from build123d import *

# Parameters (mm, degrees)
SKETCH3_R                = 1.1811
BOSS_EXTRUDE1_DEPTH      = 0.7874
BOSS_EXTRUDE1_DEPTH_BACK = 0.7874
CUT_EXTRUDE1_DEPTH       = 1.7874


with BuildPart() as part:
    # Sketch3 → Boss-Extrude1 (new body, two sides)
    with BuildSketch(Plane.XY) as boss_extrude1_sk:
        with BuildLine():
            Line((-7.084786794, -26.251475436), (-5.5626, -20.611270532))
            Line((-5.5626, -20.611270532), (-9.244241607, -19.243466133))
            ThreePointArc((-9.244241607, -19.243466133), (-11.503586026, -21.079506525), (-14.357593282, -20.504768227))
            ThreePointArc((-14.357593282, -20.504768227), (0, 22.8727), (14.357593282, -20.504768227))
            ThreePointArc((14.357593282, -20.504768227), (11.503586026, -21.079506525), (9.244241607, -19.243466133))
            Line((9.244241607, -19.243466133), (5.5626, -20.611270532))
            Line((5.5626, -20.611270532), (7.084786794, -26.251475436))
            ThreePointArc((7.084786794, -26.251475436), (0, 27.1907), (-7.084786794, -26.251475436))
        make_face()
        with Locations((-7.986421892, -21.496599331)):
            Circle(SKETCH3_R, mode=Mode.SUBTRACT)
        with Locations((7.986421892, -21.496599331)):
            Circle(SKETCH3_R, mode=Mode.SUBTRACT)
    extrude(amount=BOSS_EXTRUDE1_DEPTH)
    extrude(boss_extrude1_sk.sketch, amount=-BOSS_EXTRUDE1_DEPTH_BACK)

    # Sketch4 → Cut-Extrude1 (cut, symmetric)
    with BuildSketch(Plane.XY):
        with BuildLine():
            Line((-7.395614895, -26.165608092), (-7.395614895, -33.561222987))
            Line((-7.395614895, -33.561222987), (0, -33.561222987))
            Line((0, -33.561222987), (0, -27.1907))
            Line((0, -27.1907), (0, -20.522811972))
            Line((0, -20.522811972), (-5.800698894, -20.522811972))
            ThreePointArc((-5.800698894, -20.522811972), (-6.322313955, -23.422176045), (-7.395614895, -26.165608092))
        make_face()
    cut_extrude1 = extrude(amount=CUT_EXTRUDE1_DEPTH, both=True, mode=Mode.SUBTRACT)

    # Mirror1: Cut-Extrude1 across plane
    add(cut_extrude1.mirror(Plane(origin=(0, 0, 0), x_dir=(0, 0, 1), z_dir=(1, 0, 0))), mode=Mode.SUBTRACT)


solid = part.part
Could you check a few things on this model? Use its own coordinates, in mm. A direction names the side the tool comes from. Give positions to 0.01 mm unless a question says otherwise; leave off trailing zeros. Order: outer loops, then holes, each group sorted by start corner. A loop starts at its lowest first (then second) coordinate and runs counter-clockwise, first axis right, second up. Notation, with made-up numbers: M 48,-36.5 L 59,-36.5 A30 cw 59,2.5 Z; hole C -2,72.25 d8. An arc over 180 degrees is marked long. One line per question, with ' | ' between items.
1. I want a section at C-C (z = -0.45). List the corners of the cut face in (x, y) for me.
Results:
outline: M -14.36,-20.5 A24.06 cw long 14.36,-20.5 A3.41 cw 9.24,-19.24 L 5.8,-20.52 A15.14 ccw 7.4,-26.17 A27.19 ccw long -7.4,-26.17 A15.14 ccw -5.8,-20.52 L -9.24,-19.24 A3.41 cw Z; hole C -7.99,-21.5 d2.36; hole C 7.99,-21.5 d2.36
2. I'm going to push flat-ended pins straight in: pin 1 (5 mm diameter, centred on x = 9.5, y = 16, fed in from +Z); pin 2 (8 mm diameter, centred on x = 7.5, y = 20, fed in from +Z). Where does each tip first touch, or does it pass through?
Results:
pin 1: through | pin 2: z = 0.79
3. For faces 1 (the face through (-6.31, -23.38, 0.01)), 2 (the face through (-6.2, 22.4, 0.787)), 3 (the face through (-11.46, -21.07, 0.01)), which set-ups out of +Z, -Z, +X, -X, +Y, -Y let a thin tool reach every point of the face, with its end or its side?
Results:
face 1: +Z, -Z, -Y | face 2: +Z, +X, -X, +Y, -Y | face 3: +Z, -Z
4. If I drill on line 1 (Y direction, x = 8, z = -0.3); line 2 (Y direction, x = -0.5, z = 0.75); line 3 (X direction, y = 13.5, z = 0.75), over which ranges is the centre line in solid material (lowest first)?
Results:
line 1: -25.99 to -22.68, -20.32 to -19.71, 21.5 to 25.99 | line 2: 22.87 to 27.19 | line 3: -23.6 to -19.06, 19.06 to 23.6
5. I want a section at D-D (x = 8.5). List the corners of the cut face in (y, z) for me, and give its area (3 significant figures).
Results:
outline: M -25.83,-0.79 L -22.56,-0.79 L -22.56,0.79 L -25.83,0.79 Z; M -20.43,-0.79 L -19.52,-0.79 L -19.52,0.79 L -20.43,0.79 Z; M 21.32,-0.79 L 25.83,-0.79 L 25.83,0.79 L 21.32,0.79 Z | area: 13.7 mm²
6. I want a section at A-A (y = 0). List the corners of the cut face in (x, z) for me.
Results:
outline: M -27.19,-0.79 L -24.04,-0.79 L -24.04,0.79 L -27.19,0.79 Z; M 24.04,-0.79 L 27.19,-0.79 L 27.19,0.79 L 24.04,0.79 Z
7. We'd pull the mould along Y, two halves only. Please class faces 4 (the face through (1.09, 27.17, 0.01)), 5 (the face through (11.54, -21.09, 0.01)), 6 (the face through (6.31, -23.38, 0.01)): +Y half, -Y half, draft (parallel to the pull), parting line (faces both ways), or undercut.
Results:
face 4: parting line | face 5: undercut | face 6: -Y half
8. I want a section at B-B (x = -22.5). List the corners of the cut face in (y, z) for me.
Results:
outline: M -15.27,-0.79 L -9.73,-0.79 L -9.73,0.79 L -15.27,0.79 Z; M 7.34,-0.79 L 15.27,-0.79 L 15.27,0.79 L 7.34,0.79 Z
